```python
from build123d import *

# Parameters (mm, degrees)
SKETCH1_R           = 2.4892
BOSS_EXTRUDE2_DEPTH = 1.143
FILLET1_R           = 3.175


with BuildPart() as part:
    # Sketch1 → Boss-Extrude2 (new, symmetric)
    with BuildSketch(Plane(origin=(0, 0, 0), x_dir=(1, 0, 0), z_dir=(0, 1, 0))):
        Polygon((0, 0), (0, 152.4), (-25.4, 152.4), (-152.4, 25.4), (-152.4, 0), align=None)
        with Locations(Location((-12.7, 12.7, 0), (0, 0, 270))):
            Circle(SKETCH1_R, mode=Mode.SUBTRACT)
        with Locations(Location((-38.1, 12.7, 0), (0, 0, 270))):
            Circle(SKETCH1_R, mode=Mode.SUBTRACT)
        with Locations(Location((-63.5, 12.7, 0), (0, 0, 270))):
            Circle(SKETCH1_R, mode=Mode.SUBTRACT)
        with Locations(Location((-88.9, 12.7, 0), (0, 0, 270))):
            Circle(SKETCH1_R, mode=Mode.SUBTRACT)
        with Locations(Location((-114.3, 12.7, 0), (0, 0, 270))):
            Circle(SKETCH1_R, mode=Mode.SUBTRACT)
        with Locations(Location((-12.7, 38.1, 0), (0, 0, 270))):
            Circle(SKETCH1_R, mode=Mode.SUBTRACT)
        with Locations(Location((-12.7, 63.5, 0), (0, 0, 270))):
            Circle(SKETCH1_R, mode=Mode.SUBTRACT)
        with Locations(Location((-12.7, 88.9, 0), (0, 0, 270))):
            Circle(SKETCH1_R, mode=Mode.SUBTRACT)
        with Locations(Location((-12.7, 114.3, 0), (0, 0, 270))):
            Circle(SKETCH1_R, mode=Mode.SUBTRACT)
        with Locations(Location((-139.7, 12.7, 0), (0, 0, 270))):
            Circle(SKETCH1_R, mode=Mode.SUBTRACT)
        with Locations(Location((-12.7, 139.7, 0), (0, 0, 270))):
            Circle(SKETCH1_R, mode=Mode.SUBTRACT)
    extrude(amount=BOSS_EXTRUDE2_DEPTH, both=True)

    # Fillet1
    fillet1_edges = [part.edges().sort_by_distance(p)[0] for p in [
        (-152.4, 0, 0),
        (0, 0, 0),
    ]]
    fillet(fillet1_edges, radius=FILLET1_R)


solid = part.part
```
The model under review builds one solid part; all positions refer to its coordinate system, in mm. Round coordinates to 2 decimals unless told otherwise and drop trailing zeros. Loops run counter-clockwise (first coordinate to the right, second up) from the corner with the lowest first, then second, coordinate; pieces in that order, holes last. Notation, with made-up numbers: (-7.75, 55.25) - (16.25, 55.25) arc R10 cw to (16.25, 63.25) - close; hole circle Ø6 at (49, 76). An arc over 180 degrees is marked (long way). Use a Markdown table: item, result. Add a question column.
Q1. Add section C-C (x = -114.3). State the section outline as (y, z) points, plus the area to 3 significant figures.
Q2. The part is to be moulded in two halves that separate along Z. For faces 1 (the face through (-60, 1.143, -60)), 2 (the face through (-88, 0, -89.8)), 3 (the face through (-141.908, -0.016, -11.551)), say which applies: pulls with the +Z half, pulls with the -Z half, needs draft (parallel to the pull), parting line crosses it, or undercut.
Q3. Add section A-A (x = -12.7). State the section outline as (y, z) points.
Q4. Add section D-D (z = -12.7). State the section outline as (x, y) points, plus the area to 3 significant figures.
Q5. For probe 1 along X at (y, z) = (0.1, -63.5); probe 2 along X at (y, z) = (0.45, -138.5); probe 3 along Z at (x, y) = (-128.5, 0.15), list the stretches that pass through material, from the lowest coordinate up.
Q6. Add section B-B (z = -88.9). State the section outline as (x, y) points, plus the area to 3 significant figures.
Worked answers:
| question | item | result |
|---|---|---|
| 1 | outline | (-1.14, -63.5) - (1.14, -63.5) - (1.14, -15.19) - (-1.14, -15.19) - close; (-1.14, -10.21) - (1.14, -10.21) - (1.14, 0) - (-1.14, 0) - close |
| 1 | area | 134 mm² |
| 2 | face 1 | needs draft |
| 2 | face 2 | pulls with the -Z half |
| 2 | face 3 | undercut |
| 3 | outline | (-1.14, -152.4) - (1.14, -152.4) - (1.14, -142.19) - (-1.14, -142.19) - close; (-1.14, -137.21) - (1.14, -137.21) - (1.14, -116.79) - (-1.14, -116.79) - close; (-1.14, -111.81) - (1.14, -111.81) - (1.14, -91.39) - (-1.14, -91.39) - close; (-1.14, -86.41) - (1.14, -86.41) - (1.14, -65.99) - (-1.14, -65.99) - close; (-1.14, -61.01) - (1.14, -61.01) - (1.14, -40.59) - (-1.14, -40.59) - close; (-1.14, -35.61) - (1.14, -35.61) - (1.14, -15.19) - (-1.14, -15.19) - close; (-1.14, -10.21) - (1.14, -10.21) - (1.14, 0) - (-1.14, 0) - close |
| 4 | outline | (-152.4, -1.14) - (-142.19, -1.14) - (-142.19, 1.14) - (-152.4, 1.14) - close; (-137.21, -1.14) - (-116.79, -1.14) - (-116.79, 1.14) - (-137.21, 1.14) - close; (-111.81, -1.14) - (-91.39, -1.14) - (-91.39, 1.14) - (-111.81, 1.14) - close; (-86.41, -1.14) - (-65.99, -1.14) - (-65.99, 1.14) - (-86.41, 1.14) - close; (-61.01, -1.14) - (-40.59, -1.14) - (-40.59, 1.14) - (-61.01, 1.14) - close; (-35.61, -1.14) - (-15.19, -1.14) - (-15.19, 1.14) - (-35.61, 1.14) - close; (-10.21, -1.14) - (0, -1.14) - (0, 1.14) - (-10.21, 1.14) - close |
| 4 | area | 280 mm² |
| 5 | probe 1 | -114.3 to -15.19, -10.21 to 0 |
| 5 | probe 2 | -39.3 to -14.88, -10.52 to 0 |
| 5 | probe 3 | -49.3 to 0 |
| 6 | outline | (-88.9, -1.14) - (-15.19, -1.14) - (-15.19, 1.14) - (-88.9, 1.14) - close; (-10.21, -1.14) - (0, -1.14) - (0, 1.14) - (-10.21, 1.14) - close |
| 6 | area | 192 mm² |
